Could you check a few things on this model? Use its own coordinates, in mm. Round coordinates to 2 decimals unless told otherwise and drop trailing zeros. Loops run counter-clockwise (first coordinate to the right, second up) from the corner with the lowest first, then second, coordinate; pieces in that order, holes last. Notation, with made-up numbers: (-2.75, 27.25) -> (53.25, 27.25) arc R11 ccw to (53.25, 35.25) -> close; hole circle Ø1 at (-5, 1.5). An arc over 180 degrees is marked (long way). One line per item, written item: value.
```python
from build123d import *

# Parameters (mm, degrees)
F0_R     = 18.4
F0_R_2   = 1.4
F0_R_3   = 9
F1_DEPTH = 4
F2_R     = 1.85
F3_DEPTH = 25
F5_DEPTH = 25


with BuildPart() as f1:
    # F0 (on Front) → F1 (new body)
    with BuildSketch(Plane.XZ):
        Circle(F0_R)
        with Locations((-8.25, -11.3551508439)):
            Circle(F0_R_2, mode=Mode.SUBTRACT)
        with Locations((8.25, -11.3551508439)):
            Circle(F0_R_2, mode=Mode.SUBTRACT)
        with Locations((-13.3487804072, 4.337281675)):
            Circle(F0_R_2, mode=Mode.SUBTRACT)
        Circle(F0_R_3, mode=Mode.SUBTRACT)
        with Locations((13.3487804072, 4.337281675)):
            Circle(F0_R_2, mode=Mode.SUBTRACT)
        with Locations((0, 14.0357383378)):
            Circle(F0_R_2, mode=Mode.SUBTRACT)
    extrude(amount=-F1_DEPTH)

    # F2 (on face) → F3 (cut)
    with BuildSketch(Plane(origin=(0, 4, 0), x_dir=(-1, 0, 0), z_dir=(0, 1, 0))):
        with Locations((0, -15.4548132206)):
            Circle(F2_R)
        with Locations((13.3842608598, -7.7274066103)):
            Circle(F2_R)
        with Locations((-13.3842608598, -7.7274066103)):
            Circle(F2_R)
        with Locations((-7.7274066103, 13.3842608598)):
            Circle(F2_R)
        with Locations((7.7274066103, 13.3842608598)):
            Circle(F2_R)
    extrude(amount=-F3_DEPTH, mode=Mode.SUBTRACT)

    # F4 (on face) → F5 (cut)
    with BuildSketch(Plane.XZ):
        with BuildLine():
            ThreePointArc((-18.2913043478, -1.9970441295), (-16.9478651398, -1.3752470134), (-16.4, 0))
            ThreePointArc((-16.4, 0), (-16.9478651398, 1.3752470134), (-18.2913043478, 1.9970441295))
            ThreePointArc((-18.2913043478, 1.9970441295), (-18.4, 0), (-18.2913043478, -1.9970441295))
        make_face()
        with BuildLine():
            ThreePointArc((18.4, 0), (18.3728059915, 1), (18.2913043478, 1.9970441295))
            ThreePointArc((18.2913043478, 1.9970441295), (16.4, 0), (18.2913043478, -1.9970441295))
            ThreePointArc((18.2913043478, -1.9970441295), (18.3728059915, -1), (18.4, 0))
        make_face()
    extrude(amount=-F5_DEPTH, mode=Mode.SUBTRACT)


solid = f1.part
```
(1) We'd pull the mould along Z, two halves only. Please class faces 1 (the face through (0.377, 1.972, 18.396)), 2 (the face through (-0.377, 1.972, -18.396)), 3 (the face through (-8.553, 1.972, -12.722)): +Z half, -Z half, draft (parallel to the pull), parting line (faces both ways), or undercut.
Results below:
face 1: +Z half
face 2: -Z half
face 3: undercut
(2) Please list where these lines run through material, in increasing order: L1, parallel to Z at x = 0, y = 2.15; L2, parallel to X at y = 1, z = 4; L3, parallel to Z at x = 7, y = 0.65.
Results below:
L1: z = -18.4 to -17.3, -13.6 to -9, 9 to 12.64, 15.44 to 18.4
L2: x = -17.96 to -14.71, -11.99 to -8.06, 8.06 to 11.99, 14.71 to 17.96
L3: z = -17.02 to -11.99, -10.72 to -5.66, 5.66 to 11.68, 15.09 to 17.02
(3) Imagine slicing it at B-B on y = 2.85. Give the number of separate pieces and of enclosed holes in the cut face, then the cut area to 3 significant figures.
Results below:
separate pieces: 1
enclosed holes: 11
area: 712 mm²
(4) Imagine slicing it at D-D on x = 13. Write out the boundary of the cut face in (y, z), then the cut area to 3 significant figures.
Results below:
outline: (0, -13.02) -> (4, -13.02) -> (4, -9.54) -> (0, -9.54) -> close; (0, -5.92) -> (4, -5.92) -> (4, 2.98) -> (0, 2.98) -> close; (0, 5.69) -> (4, 5.69) -> (4, 13.02) -> (0, 13.02) -> close
area: 78.8 mm²
(5) For pin 1 Ø1 at (x, y) = (12, 3) entering from +Z, with a flat end and sliding along its axis, tell me the tip position at first contact or that it passes through.
Results below:
pin 1: stops at z = 14.36
(6) Imagine slicing it at C-C on z = -8.5. Write out the boundary of the cut face in (x, y), then the cut area to 3 significant figures.
Results below:
outline: (-16.32, 0) -> (-15.07, 0) -> (-15.07, 4) -> (-16.32, 4) -> close; (-11.7, 0) -> (-2.96, 0) -> (-2.96, 4) -> (-11.7, 4) -> close; (2.96, 0) -> (11.7, 0) -> (11.7, 4) -> (2.96, 4) -> close; (15.07, 0) -> (16.32, 0) -> (16.32, 4) -> (15.07, 4) -> close
area: 80.0 mm²
(7) Imagine slicing it at A-A on x = 0. Write out the boundary of the cut face in (y, z).
Results below:
outline: (0, -18.4) -> (4, -18.4) -> (4, -17.3) -> (0, -17.3) -> close; (0, -13.6) -> (4, -13.6) -> (4, -9) -> (0, -9) -> close; (0, 9) -> (4, 9) -> (4, 12.64) -> (0, 12.64) -> close; (0, 15.44) -> (4, 15.44) -> (4, 18.4) -> (0, 18.4) -> close
